Part model, mm, in its own coordinate system. A direction names the side the tool comes from. Coordinates: 2 decimals unless noted, no trailing zeros. Order: outer loops, then holes, each group sorted by start corner. A loop starts at its lowest first (then second) coordinate and runs counter-clockwise, first axis right, second up. Notation, with made-up numbers: (28.25, 86.25) - (38.25, 86.25) arc R29 cw to (38.25, 114.25) - close; hole circle Ø5 at (25.25, 86.5). An arc over 180 degrees is marked (long way). Use a Markdown table: item, result. Add a question column.
1) Saw through at A-A on z = 0.75. List the corners of the cut face in (x, y) (3 decimals).
2) Saw through at B-B on y = -6. List the corners of the cut face in (x, z).
3) Tool access for faces 1 (the face through (14, -4, 1)), 2 (the face through (-14.26, -12.31, 1.01)): list every direction of +Z, -Z, +X, -X, +Y, -Y with a clear straight run to the whole face (end or side of a thin tool).
4) Saw through at D-D on y = -13. List the corners of the cut face in (x, z) (3 decimals).
5) Wall check: L1, parallel to Y at x = -7, z = 1.65; L2, parallel to Y at x = -8.5, z = 0.85 (3 decimals); L3, parallel to Y at x = -3.5, z = 0.7 (1 decimal). Give the ranges that are in metal, low to high. Write a range as [from, to].
6) Saw through at C-C on x = -10. List the corners of the cut face in (y, z).
7) Drop flat-ended pins along their axis: P1, Ø2.5, axis at x = -3.5, y = -13, coming from the +Z side; P2, Ø1.9, axis at x = 12.5, y = 0, coming from the -Z side; P3, Ø0.6, axis at x = 16, z = 0.5, coming from the -Y side. Give the stop position or say it passes through.
```python
from build123d import *

# Parameters (mm, degrees)
SKETCH_2_W          = 31
SKETCH_2_H          = 8
EXTRUDE_1_DEPTH     = 2
SKETCH_3_R          = 1.55
CUT_EXTRUDE_1_DEPTH = 2
SKETCH_4_W          = 4
SKETCH_4_H          = 12
EXTRUDE_2_DEPTH     = 2
SKETCH_5_R          = 1.025
CUT_EXTRUDE_2_DEPTH = 2
SKETCH_6_W          = 9
SKETCH_6_H          = 8
EXTRUDE_3_DEPTH     = 2
FILLET_1_R          = 2
EXTRUDE_START       = -2
EXTRUDE_4_OUTLINE_R = 1.025
EXTRUDE_4_DEPTH     = 2
FILLET_2_R          = 5
SKETCH_8_R          = 4
CUT_EXTRUDE_3_DEPTH = 2


# Read off the part's stored shape, not the designer's step: 凸台-拉伸4
with BuildPart() as part:
    # 草图2 → 凸台-拉伸1 (new body)
    with BuildSketch(Plane.XY):
        Rectangle(SKETCH_2_W, SKETCH_2_H)
    extrude(amount=EXTRUDE_1_DEPTH)

    # 草图3 → 切除-拉伸1 (cut)
    with BuildSketch(Plane.XY.offset(2)):
        with Locations((12.5, 0)):
            Circle(SKETCH_3_R)
        with Locations((-12.5, 0)):
            Circle(SKETCH_3_R)
    extrude(amount=-CUT_EXTRUDE_1_DEPTH, mode=Mode.SUBTRACT)

    # 草图4 → 凸台-拉伸2 (add)
    with BuildSketch(Plane.XY.offset(2)):
        with Locations((-13.5, -10)):
            Rectangle(SKETCH_4_W, SKETCH_4_H)
    extrude(amount=-EXTRUDE_2_DEPTH)

    # 草图5 → 切除-拉伸2 (cut)
    with BuildSketch(Plane.XY.offset(2)):
        with Locations((-13.5, -13)):
            Circle(SKETCH_5_R)
    extrude(amount=-CUT_EXTRUDE_2_DEPTH, mode=Mode.SUBTRACT)

    # 草图6 → 凸台-拉伸3 (add)
    with BuildSketch(Plane.XY.offset(2)):
        with Locations((20, 0)):
            Rectangle(SKETCH_6_W, SKETCH_6_H)
    extrude(amount=-EXTRUDE_3_DEPTH)

    # 圆角1
    fillet_1_edges = [part.edges().sort_by_distance(p)[0] for p in [
        (-15.5, -16, 1),
        (-11.5, -16, 1),
        (-11.5, -4, 1),
        (-15.5, 4, 1),
        (24.5, -4, 1),
        (24.5, 4, 1),
    ]]
    fillet(fillet_1_edges, radius=FILLET_1_R - 0.0001)  # a hair under: the kernel refuses the full size

    # 凸台-拉伸4 outline → 凸台-拉伸4 (add)
    with BuildSketch(Plane.XY.offset(2).offset(EXTRUDE_START)):
        with BuildLine():
            Line((-13.5, -16), (0, -16))
            Line((0, -16), (0, -4))
            Line((0, -4), (-11.499999994, -4))
            Line((-11.499999994, -4), (-11.5, -14))
            ThreePointArc((-11.5, -14), (-12.085786438, -15.414213562), (-13.5, -16))
        make_face()
        with Locations((-8.5, -13)):
            Circle(EXTRUDE_4_OUTLINE_R, mode=Mode.SUBTRACT)
        with Locations((-3.5, -13)):
            Circle(EXTRUDE_4_OUTLINE_R, mode=Mode.SUBTRACT)
    extrude(amount=EXTRUDE_4_DEPTH)

    # 圆角2
    fillet_2_edges = [part.edges().sort_by_distance(p)[0] for p in [
        (0, -4, 1),
        (0, -16, 1),
    ]]
    fillet(fillet_2_edges, radius=FILLET_2_R)

    # 草图8 → 切除-拉伸3 (cut)
    with BuildSketch(Plane.XY.offset(2)):
        with Locations((-7, -6)):
            Circle(SKETCH_8_R)
    extrude(amount=-CUT_EXTRUDE_3_DEPTH, mode=Mode.SUBTRACT)


solid = part.part
```
Results are:
| question | item | result |
|---|---|---|
| 1 | outline | (-15.5, -14) arc R2 ccw to (-13.5, -16) - (-5, -16) arc R5 ccw to (0, -11) - (0, -9) arc R5 cw to (5, -4) - (22.5, -4) arc R2 ccw to (24.5, -2) - (24.5, 2) arc R2 ccw to (22.5, 4) - (-13.5, 4) arc R2 ccw to (-15.5, 2) - close; hole circle Ø2.05 at (-13.5, -13); hole circle Ø3.1 at (-12.5, 0); hole circle Ø8 at (-7, -6); hole circle Ø2.05 at (-8.5, -13); hole circle Ø2.05 at (-3.5, -13); hole circle Ø3.1 at (12.5, 0) |
| 2 | outline | (-15.5, 0) - (-11, 0) - (-11, 2) - (-15.5, 2) - close; (-3, 0) - (1, 0) - (1, 2) - (-3, 2) - close |
| 3 | face 1 | +Z, -Z, +X, -Y |
| 3 | face 2 | +Z, -Z |
| 4 | outline | (-15.5, 0) - (-14.525, 0) - (-14.525, 2) - (-15.5, 2) - close; (-12.475, 0) - (-9.525, 0) - (-9.525, 2) - (-12.475, 2) - close; (-7.475, 0) - (-4.525, 0) - (-4.525, 2) - (-7.475, 2) - close; (-2.475, 0) - (-0.417, 0) - (-0.417, 2) - (-2.475, 2) - close |
| 5 | L1 | [-16, -10], [-2, 4] |
| 5 | L2 | [-16, -14.025], [-11.975, -9.708], [-2.292, 4] |
| 5 | L3 | [-15.8, -14], [-12, -7.9], [-4.1, 4] |
| 6 | outline | (-16, 0) - (-8.65, 0) - (-8.65, 2) - (-16, 2) - close; (-3.35, 0) - (4, 0) - (4, 2) - (-3.35, 2) - close |
| 7 | P1 | z = 2 |
| 7 | P2 | through |
| 7 | P3 | y = -4 |
